from build123d import *

# Parameters (mm, degrees)
PAD_DEPTH = 19


with BuildPart() as part:
    # Sketch → Pad (new body)
    with BuildSketch(Plane.XY):
        with BuildLine():
            Line((0, 0), (-60, 0))
            ThreePointArc((-60, 0), (-75, -15), (-60, -30))
            Line((-60, -30), (-23.5, -30))
            ThreePointArc((-23.5, -30), (-18.903806, -28.096194), (-17, -23.5))
            ThreePointArc((0, -23.5), (-8.5, -15), (-17, -23.5))
            Line((0, -23.5), (-2, -23.5))
            ThreePointArc((-2, -23.5), (-8.5, -17), (-15, -23.5))
            ThreePointArc((-23.5, -32), (-17.489592, -29.510408), (-15, -23.5))
            Line((-60, -32), (-23.5, -32))
            ThreePointArc((-60, 2), (-77, -15), (-60, -32))
            Line((-60, 2), (0, 2))
            Line((0, 2), (0, 0))
        make_face()
    extrude(amount=PAD_DEPTH)


solid = part.part
The model under review builds one solid part; all positions refer to its coordinate system, in mm. A direction names the side the tool comes from. Give positions to 0.01 mm unless a question says otherwise; leave off trailing zeros. Order: outer loops, then holes, each group sorted by start corner. A loop starts at its lowest first (then second) coordinate and runs counter-clockwise, first axis right, second up. Notation, with made-up numbers: M -12.75,-32.5 L -6.75,-32.5 A18 ccw -6.75,-8.5 Z; hole C 29.5,-21 d3. An arc over 180 degrees is marked long. Use one line per item in the form item = value. Start each with the question number.
Item 1: To check wall thickness, follow line 1 along Y through (x, z) = (-50, 17.5); line 2 along X through (y, z) = (-20.5, 9.5); line 3 along X through (y, z) = (-22, 5). State the ranges of each line that lie inside material, in increasing order. Write a range as from..to.
Item 2: We need section D-D on x = -5. Give the boundary of the cut face in (y, z), plus the area to 3 significant figures.
Item 3: We need section B-B on z = 6. Give the boundary of the cut face in (x, y).
Item 4: Insertion check: pin 1 Ø1.5 at (y, z) = (-9.5, 2) entering from -X; pin 2 Ø10 at (y, z) = (-9, 13) entering from +X; pin 3 Ø1 at (x, z) = (-16, 11.5) entering from -Y. Each pin has a flat end and moves straight along its axis. Give the tip position at first contact, or say it passes through.
Item 5: We need section A-A on x = -54. Give the boundary of the cut face in (y, z), plus the area to 3 significant figures.
Item 6: For faces 5 (the flat face through (-1, -23.5, 9)), 6 (the cylindrical face through (-18.955, -28.146, 9.367)), 7 (the flat face through (-41.2, 0.2, 19)), list the 3-axis set-ups (+Z, -Z, +X, -X, +Y, -Y) from which the entire face can be reached by the end or side of a thin tool; tool diameter is ignored.
Item 7: The part is to be moulded in two halves that separate along Y. For faces 1 (the flat face through (-30, 0, 9)), 2 (the cylindrical face through (-77, -15, 9)), 3 (the cylindrical face through (-8.313, -15.002, 9.367)), 4 (the cylindrical face through (-17.56, -29.58, 9.37)), say which applies: pulls with the +Y half, pulls with the -Y half, needs draft (parallel to the pull), parting line crosses it, or undercut.
Item 8: We need section C-C on y = -20.5. Give the boundary of the cut face in (x, z), plus the area to 3 significant figures.
Completed:
q1.line_1 = -32..-30, 0..2
q1.line_2 = -76.09..-73.96, -16.45..-14.27, -2.73..-0.55
q1.line_3 = -75.49..-73.27, -16.87..-14.82, -2.18..-0.13
q2.outline = M -18.02,0 L -15.75,0 L -15.75,19 L -18.02,19 Z; M 0,0 L 2,0 L 2,19 L 0,19 Z
q2.area = 81.1 mm²
q3.outline = M -60,-32 L -23.5,-32 A8.5 ccw -15,-23.5 A6.5 cw -2,-23.5 L 0,-23.5 A8.5 ccw -17,-23.5 A6.5 cw -23.5,-30 L -60,-30 A15 cw -60,0 L 0,0 L 0,2 L -60,2 A17 ccw Z
q4.pin_1 = -76.32
q4.pin_2 = -70.2
q4.pin_3 = -28.32
q5.outline = M -32,0 L -30,0 L -30,19 L -32,19 Z; M 0,0 L 2,0 L 2,19 L 0,19 Z
q5.area = 76.0 mm²
q6.face_5 = +Z, -Z, +X, -Y
q6.face_6 = +Z, -Z
q6.face_7 = +Z, +X, -X, +Y, -Y
q7.face_1 = undercut
q7.face_2 = parting line crosses it
q7.face_3 = undercut
q7.face_4 = pulls with the -Y half
q8.outline = M -76.09,0 L -73.96,0 L -73.96,19 L -76.09,19 Z; M -16.45,0 L -14.27,0 L -14.27,19 L -16.45,19 Z; M -2.73,0 L -0.55,0 L -0.55,19 L -2.73,19 Z
q8.area = 124 mm²
